from build123d import *

# Parameters (mm, degrees)
SKETCH_1_W          = 32
SKETCH_1_H          = 32
SKETCH_1_R          = 1.65
EXTRUDE_1_DEPTH     = 2
SKETCH_2_W          = 18
SKETCH_2_H          = 26
CUT_EXTRUDE_1_DEPTH = 23.715633383
FILLET_1_R          = 2


with BuildPart() as part:
    # 草图1 → 凸台-拉伸1 (new body)
    with BuildSketch(Plane(origin=(0, 0, 0), x_dir=(1, 0, 0), z_dir=(0, 1, 0))):
        Rectangle(SKETCH_1_W, SKETCH_1_H)
        with Locations(Location((-12.75, 12.75, 0), (0, 0, 270))):
            Circle(SKETCH_1_R, mode=Mode.SUBTRACT)
        with Locations(Location((12.75, 12.75, 0), (0, 0, 90))):
            Circle(SKETCH_1_R, mode=Mode.SUBTRACT)
        with Locations(Location((12.75, -12.75, 0), (0, 0, 270))):
            Circle(SKETCH_1_R, mode=Mode.SUBTRACT)
        with Locations(Location((-12.75, -12.75, 0), (0, 0, 90))):
            Circle(SKETCH_1_R, mode=Mode.SUBTRACT)
        with Locations(Location((-12.15, 6, 0), (0, 0, 270))):
            Circle(SKETCH_1_R, mode=Mode.SUBTRACT)
        with Locations(Location((-12.15, -6, 0), (0, 0, 90))):
            Circle(SKETCH_1_R, mode=Mode.SUBTRACT)
        with Locations(Location((12.15, -6, 0), (0, 0, 270))):
            Circle(SKETCH_1_R, mode=Mode.SUBTRACT)
        with Locations(Location((12.15, 6, 0), (0, 0, 90))):
            Circle(SKETCH_1_R, mode=Mode.SUBTRACT)
    extrude(amount=EXTRUDE_1_DEPTH)

    # 草图2 → 切除-拉伸1 (cut, through all)
    with BuildSketch(Plane(origin=(0, 2, 0), x_dir=(1, 0, 0), z_dir=(0, 1, 0))):
        Rectangle(SKETCH_2_W, SKETCH_2_H)
    extrude(amount=-CUT_EXTRUDE_1_DEPTH, mode=Mode.SUBTRACT)

    # 圆角1
    fillet_1_edges = [part.edges().sort_by_distance(p)[0] for p in [
        (-9, 1, 13),
        (-9, 1, -13),
        (9, 1, -13),
        (9, 1, 13),
        (16, 1, 16),
        (-16, 1, 16),
        (-16, 1, -16),
        (16, 1, -16),
    ]]
    fillet(fillet_1_edges, radius=FILLET_1_R)


solid = part.part
Input: part model. Units: mm. Frame: model coordinates. A direction names the side the tool comes from. Give positions to 0.01 mm unless a question says otherwise; leave off trailing zeros. Order: outer loops, then holes, each group sorted by start corner. A loop starts at its lowest first (then second) coordinate and runs counter-clockwise, first axis right, second up.
Q1. Section D-D on z = -6. Output: boundary loops of the cut face in (x, y), and give its area (3 significant figures).
Checked values:
outline: (-16, 0) - (-13.8, 0) - (-13.8, 2) - (-16, 2) - close; (-10.5, 0) - (-9, 0) - (-9, 2) - (-10.5, 2) - close; (9, 0) - (10.5, 0) - (10.5, 2) - (9, 2) - close; (13.8, 0) - (16, 0) - (16, 2) - (13.8, 2) - close
area: 14.8 mm2
Q2. Section C-C on y = 0.6. State how many separate pieces and enclosed holes the cut face has, and give its area (3 significant figures).
Checked values:
separate pieces: 1
enclosed holes: 9
area: 488 mm2
Q3. Set-up query: faces 5 (the flat face through (0, 1, -13)), 6 (the cylindrical face through (-15.43, 1.01, -15.4)). Return all of +Z, -Z, +X, -X, +Y, -Y with unobstructed straight access to the full face (end or side cutting, diameter ignored); none if empty.
Checked values:
face 5: +Y, -Y
face 6: -Z, -X, +Y, -Y
Q4. Draft query along Z for faces 1 (the flat face through (-16, 1, 0)), 2 (the cylindrical face through (13.76, 0.99, -5.64)), 3 (the cylindrical face through (15.4, 1.01, 15.43)), 4 (the flat face through (0, 1, -16)). Return one class per face: +Z half, -Z half, draft (parallel to the pull), parting line (faces both ways), or undercut.
Checked values:
face 1: draft
face 2: undercut
face 3: +Z half
face 4: -Z half
Q5. Contact query for flat-ended pins moving along their axis: pin 1 Ø2.5 at (x, z) = (-12.15, -6) entering from +Y; pin 2 Ø10 at (x, z) = (-12.5, 0) entering from -Y. Output: stop coordinate, or through.
Checked values:
pin 1: passes through
pin 2: stops at y = 0
Q6. Ray query, probe 1 along X at (y, z) = (1.7, 6); probe 2 along Z at (x, y) = (1.5, 1.3); probe 3 along X at (y, z) = (1.5, 12.75). Return the intervals inside material, ascending.
Checked values:
probe 1: x = -16 to -13.8, -10.5 to -9, 9 to 10.5, 13.8 to 16
probe 2: z = -16 to -13, 13 to 16
probe 3: x = -16 to -14.4, -11.1 to -7.97, 7.97 to 11.1, 14.4 to 16
Q7. Section A-A on x = 6. Output: boundary loops of the cut face in (y, z).
Checked values:
outline: (0, -16) - (2, -16) - (2, -13) - (0, -13) - close; (0, 13) - (2, 13) - (2, 16) - (0, 16) - close
Q8. Section B-B on z = 3.5. Output: boundary loops of the cut face in (x, y).
Checked values:
outline: (-16, 0) - (-9, 0) - (-9, 2) - (-16, 2) - close; (9, 0) - (16, 0) - (16, 2) - (9, 2) - close
